```python
from build123d import *

# Parameters (mm, degrees)
SKETCH1_R           = 10
BOSS_EXTRUDE1_DEPTH = 30
CUT_EXTRUDE1_DEPTH  = 25
FILLET1_R           = 5


with BuildPart() as part:
    # Sketch1 → Boss-Extrude1 (new body)
    with BuildSketch(Plane(origin=(0, 0, 0), x_dir=(1, 0, 0), z_dir=(0, 1, 0))):
        with BuildLine():
            Line((-90, 0), (-90, 43.954606061))
            ThreePointArc((-90, 43.954606061), (-87.507512185, 53.62347451), (-80.651298291, 60.88238928))
            Line((-80.651298291, 60.88238928), (-10.651298291, 104.927783219))
            ThreePointArc((-10.651298291, 104.927783219), (0, 108), (10.651298291, 104.927783219))
            Line((10.651298291, 104.927783219), (80.651298291, 60.88238928))
            ThreePointArc((80.651298291, 60.88238928), (87.507512185, 53.62347451), (90, 43.954606061))
            Line((90, 43.954606061), (90, 0))
            ThreePointArc((90, 0), (81.952286093, -16.035674515), (64.285714286, -19.16629695))
            Line((64.285714286, -19.16629695), (14.285714286, -4.2591771))
            ThreePointArc((14.285714286, -4.2591771), (0, -2.174919475), (-14.285714286, -4.2591771))
            Line((-14.285714286, -4.2591771), (-64.285714286, -19.16629695))
            ThreePointArc((-64.285714286, -19.16629695), (-81.952286093, -16.035674515), (-90, 0))
        make_face()
        with Locations(Location((0, 88, 0), (0, 0, 270))):
            Circle(SKETCH1_R, mode=Mode.SUBTRACT)
        with Locations(Location((-70, 0, 0), (0, 0, 270))):
            Circle(SKETCH1_R, mode=Mode.SUBTRACT)
        with Locations(Location((70, 0, 0), (0, 0, 90))):
            Circle(SKETCH1_R, mode=Mode.SUBTRACT)
    extrude(amount=BOSS_EXTRUDE1_DEPTH)

    # Sketch2 → Cut-Extrude1 (cut)
    with BuildSketch(Plane(origin=(0, 30, 0), x_dir=(1, 0, 0), z_dir=(0, 1, 0))):
        with BuildLine():
            Line((-12.013853927, 96.981498418), (-77.455908804, 55.804054314))
            ThreePointArc((-77.455908804, 55.804054314), (-82.25525853, 50.722813975), (-84, 43.954606061))
            Line((-84, 43.954606061), (-84, 5.385164807))
            ThreePointArc((-84, 5.385164807), (-61.03578543, 12.026755886), (-60.839316609, -11.877789349))
            Line((-60.839316609, -11.877789349), (-16, 1.490711985))
            ThreePointArc((-16, 1.490711985), (0, 3.825080525), (16, 1.490711985))
            Line((16, 1.490711985), (60.839316609, -11.877789349))
            ThreePointArc((60.839316609, -11.877789349), (61.03578543, 12.026755886), (84, 5.385164807))
            Line((84, 5.385164807), (84, 43.954606061))
            ThreePointArc((84, 43.954606061), (82.25525853, 50.722813975), (77.455908804, 55.804054314))
            Line((77.455908804, 55.804054314), (12.013853927, 96.981498418))
            ThreePointArc((12.013853927, 96.981498418), (0, 73), (-12.013853927, 96.981498418))
        make_face()
    extrude(amount=-CUT_EXTRUDE1_DEPTH, mode=Mode.SUBTRACT)

    # Fillet1
    fillet1_edges = [part.edges().sort_by_distance(p)[0] for p in [
        (84, 17.5, -5.385164807),
        (60.839316609, 17.5, 11.877789349),
        (-60.839316609, 17.5, 11.877789349),
        (-84, 17.5, -5.385164807),
        (-12.013853927, 17.5, -96.981498418),
        (12.013853927, 17.5, -96.981498418),
    ]]
    fillet(fillet1_edges, radius=FILLET1_R)


solid = part.part
```
Source: CAD feature listing. Evaluate the final solid. Frame: model axes, mm. A direction names the side the tool comes from. Give positions to 0.01 mm unless a question says otherwise; leave off trailing zeros. Loops run counter-clockwise (first coordinate to the right, second up) from the corner with the lowest first, then second, coordinate; pieces in that order, holes last. Notation, with made-up numbers: (42.5, -17.75) -> (92.5, -17.75) arc R14 cw to (92.5, -6.75) -> close; hole circle Ø11 at (-16.5, 1). An arc over 180 degrees is marked (long way). Put each result on its own line as item: value. Start each with the question number.
1) Reachability of faces 4 (the face through (-38.94, 14.79, 11.61)), 5 (the face through (32.212, 17.675, 3.343)), 6 (the face through (79.76, 14.79, 2.17)) from +Z, -Z, +X, -X, +Y, -Y: full face, straight path, thin tool, end or side. Return the list, or none.
2) Contact query for flat-ended pins moving along their axis: P1, Ø5, axis at y = 4, z = -79.5, coming from the -X side; P2, Ø5, axis at x = 4.5, y = 8, coming from the -Z side; P3, Ø6, axis at y = 3, z = -80.5, coming from the +X side. Output: stop coordinate, or through.
3) Cut plane D-D (x = 70). Return loops of the section in (y, z), then the cut area to 3 significant figures.
4) Cut plane C-C (z = -22.5). Return loops of the section in (x, y), then the cut area to 3 significant figures.
5) Draft query along Z for faces 1 (the face through (0, 15, -98)), 2 (the face through (39.64, 14.79, 11.82)), 3 (the face through (87.439, 14.79, -53.747)). Return one class per face: released by +Z, released by -Z, zero draft, split by the parting line, or undercut.
6) Cut plane B-B (y = 11.25). State how many separate pieces and enclosed holes the cut face has, then the cut area to 3 significant figures.
7) Cut plane A-A (x = 0). Return loops of the section in (y, z), then the cut area to 3 significant figures.
8) Material intervals for probe 1 along Z at (x, y) = (-65.5, 18); probe 2 along X at (y, z) = (6.75, -75); probe 3 along Y at (x, z) = (-28.5, -38.5), sorted ascending.
Results are:
1. face 4: +Z, +Y, -Y
1. face 5: +Y
1. face 6: +Y, -Y
2. P1: stops at x = -55.04
2. P2: stops at z = -107.9
2. P3: stops at x = 54.24
3. outline: (0, -67.58) -> (30, -67.58) -> (30, -60.5) -> (5, -60.5) -> (5, -15) -> (30, -15) -> (30, -10) -> (0, -10) -> close; (0, 10) -> (30, 10) -> (30, 20) -> (0, 20) -> close
3. area: 890 mm2
4. outline: (-90, 0) -> (90, 0) -> (90, 30) -> (84, 30) -> (84, 5) -> (-84, 5) -> (-84, 30) -> (-90, 30) -> close
4. area: 1,200 mm2
5. face 1: undercut
5. face 2: released by +Z
5. face 3: released by -Z
6. separate pieces: 1
6. enclosed holes: 4
6. area: 4,260 mm2
7. outline: (0, -108) -> (30, -108) -> (30, -98) -> (0, -98) -> close; (0, -78) -> (30, -78) -> (30, -73) -> (5, -73) -> (5, -3.83) -> (30, -3.83) -> (30, 2.17) -> (0, 2.17) -> close
7. area: 976 mm2
8. probe 1: z = -70.42 to -63.33, -14.31 to -8.93, 8.93 to 19.49
8. probe 2: x = -58.21 to -46.95, -7.48 to 7.48, 46.95 to 58.21
8. probe 3: y = 0 to 5
